```python
from build123d import *

# Parameters (mm, degrees)
F0_R     = 1
F1_DEPTH = 1.5
F3_DEPTH = 1.5
F4_DEPTH = 5
F2_W     = 4.5
F2_H     = 4.5
F2_R     = 1
F5_DEPTH = 3.5


with BuildPart() as f1:
    # F0 (on Top) → F1 (new body)
    with BuildSketch(Plane.XY):
        with BuildLine():
            ThreePointArc((-20.5, 0), (-21.232233047, 1.767766953), (-23, 2.5))
            ThreePointArc((-23, 2.5), (-25.5, 0), (-23, -2.5))
            ThreePointArc((-23, -2.5), (-21.232233047, -1.767766953), (-20.5, 0))
        make_face()
        with Locations((-23, 0)):
            Circle(F0_R, mode=Mode.SUBTRACT)
        with BuildLine():
            Line((23, 2.5), (-23, 2.5))
            ThreePointArc((-23, 2.5), (-21.232233047, 1.767766953), (-20.5, 0))
            ThreePointArc((-20.5, 0), (-21.232233047, -1.767766953), (-23, -2.5))
            Line((-23, -2.5), (23, -2.5))
            ThreePointArc((23, -2.5), (20.5, 0), (23, 2.5))
        make_face()
        with BuildLine():
            ThreePointArc((25.5, 0), (24.767766953, 1.767766953), (23, 2.5))
            ThreePointArc((23, 2.5), (20.5, 0), (23, -2.5))
            ThreePointArc((23, -2.5), (24.767766953, -1.767766953), (25.5, 0))
        make_face()
        with Locations((23, 0)):
            Circle(F0_R, mode=Mode.SUBTRACT)
    extrude(amount=F1_DEPTH)

    # F2 (on face) → F3 (join)
    with BuildSketch(Plane.XZ.offset(2.5)):
        Polygon((8.2, 37.7), (-8.2, 37.7), (-8.2, 33.2), (-12.7, 33.2), (-12.7, 25.25), (-8.2, 25.25), (-8.2, 20.75), (-12.7, 20.75), (-12.7, 13.3), (-8.25, 13.3), (-8.25, 11.8), (-12.7, 11.8), (-12.7, 1.5), (12.7, 1.5), (12.7, 11.8), (8.25, 11.8), (8.25, 13.3), (12.7, 13.3), (12.7, 20.75), (8.2, 20.75), (8.2, 25.25), (12.7, 25.25), (12.7, 33.2), (8.2, 33.2), align=None)
        Polygon((-6.5, 27.5), (-4.5, 27.5), (4.5, 27.5), (6.5, 27.5), (6.5, 16.5), (-6.5, 16.5), align=None, mode=Mode.SUBTRACT)
    extrude(amount=-F3_DEPTH)

    # F2 (on face) → F4 (join)
    with BuildSketch(Plane.XZ.offset(2.5)):
        Polygon((-12.7, 33.2), (-12.7, 37.7), (-8.2, 37.7), (8.2, 37.7), (12.7, 37.7), (12.7, 33.2), (12.7, 25.25), (12.7, 20.75), (12.7, 13.3), (8.25, 13.3), (8.25, 11.8), (12.7, 11.8), (12.7, 1.5), (14.2, 1.5), (14.2, 39.2), (-14.2, 39.2), (-14.2, 1.5), (-12.7, 1.5), (-12.7, 11.8), (-8.25, 11.8), (-8.25, 13.3), (-12.7, 13.3), (-12.7, 20.75), (-12.7, 25.25), align=None)
    extrude(amount=-F4_DEPTH)

    # F2 (on face) → F5 (join)
    with BuildSketch(Plane.XZ.offset(2.5)):
        with Locations((10.45, 35.45)):
            Rectangle(F2_W, F2_H)
        with Locations((10.5, 35.5)):
            Circle(F2_R, mode=Mode.SUBTRACT)
        with Locations((10.45, 23)):
            Rectangle(F2_W, F2_H)
        with Locations((10.5, 23)):
            Circle(F2_R, mode=Mode.SUBTRACT)
        Polygon((-4.5, 18.5), (-4.5, 27.5), (-6.5, 27.5), (-6.5, 16.5), (6.5, 16.5), (6.5, 27.5), (4.5, 27.5), (4.5, 18.5), align=None)
        with Locations((-10.45, 35.45)):
            Rectangle(F2_W, F2_H)
        with Locations((-10.5, 35.5)):
            Circle(F2_R, mode=Mode.SUBTRACT)
        with Locations((-10.45, 23)):
            Rectangle(F2_W, F2_H)
        with Locations((-10.5, 23)):
            Circle(F2_R, mode=Mode.SUBTRACT)
    extrude(amount=-F5_DEPTH)


solid = f1.part
```
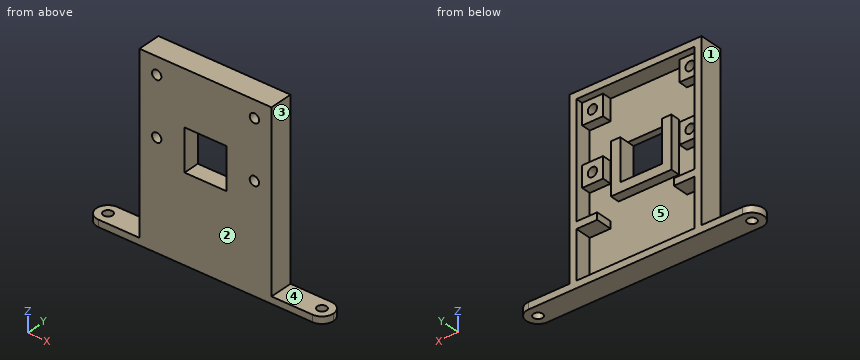
Geometry check sheet. Reference: the model listing, model coordinates, mm. Face numbers are marked on the shaded views. A direction names the side the tool comes from. Give positions to 0.01 mm unless a question says otherwise; leave off trailing zeros. Order: outer loops, then holes, each group sorted by start corner. A loop starts at its lowest first (then second) coordinate and runs counter-clockwise, first axis right, second up. Notation, with made-up numbers: (34.5, 32) -> (67.5, 32) arc R28 cw to (67.5, 68) -> close; hole circle Ø11 at (-14, 52). An arc over 180 degrees is marked (long way). Write each question's results on one line, items separated by ' | '. Start each with the question number.
(1) Sectioned sample at A-A (z = 23). Enter the section's corners in (x, y).
(2) Sectioned sample at C-C (x = 10.5). Enter the section's corners in (y, z), plus the area to 4 significant figures.
(3) Scan lines: line 1 (Z direction, x = -12, y = -0.3); line 2 (Z direction, x = -4, y = 0.65); line 3 (X direction, y = -0.05, z = 17). Record each from-to range of solid material in increasing order.
(4) Sectioned sample at D-D (z = 32). Enter the section's corners in (x, y), plus the area to 3 significant figures.
(5) Gauge pin test, flat ends, axial feed: P1, Ø2.5, axis at x = -10.5, z = 23, coming from the +Y side; P2, Ø1.8, axis at y = 0.5, z = 9, coming from the +X side; P3, Ø1, axis at y = -0.5, z = 22.5, coming from the -X side; P4, Ø1.6, axis at x = 23, y = 0, coming from the -Z side. Record the tip position at first contact, or that the pin passes through.
(6) Access from +Z, -Z, +X, -X, +Y, -Y to the whole of each face (thin tool, end or side, straight path). Record for the marked faces 1 and 2.
(7) Mould release check, pull along X, two halves, no side actions. Record for the marked faces 3, 4 and 5: pulls with the +X half, pulls with the -X half, needs draft (parallel to the pull), parting line crosses it, or undercut.
(8) Sectioned sample at B-B (x = 3.5). Enter the section's corners in (y, z).
Answer below:
1) outline: (-14.2, -2.5) -> (-11.5, -2.5) -> (-11.5, 1) -> (-12.7, 1) -> (-12.7, 2.5) -> (-14.2, 2.5) -> close; (-9.5, -2.5) -> (-4.5, -2.5) -> (-4.5, 1) -> (-6.5, 1) -> (-6.5, -1) -> (-8.2, -1) -> (-8.2, 1) -> (-9.5, 1) -> close; (4.5, -2.5) -> (9.5, -2.5) -> (9.5, 1) -> (8.2, 1) -> (8.2, -1) -> (6.5, -1) -> (6.5, 1) -> (4.5, 1) -> close; (11.5, -2.5) -> (14.2, -2.5) -> (14.2, 2.5) -> (12.7, 2.5) -> (12.7, 1) -> (11.5, 1) -> close
2) outline: (-2.5, 0) -> (2.5, 0) -> (2.5, 1.5) -> (-1, 1.5) -> (-1, 11.8) -> (2.5, 11.8) -> (2.5, 13.3) -> (-1, 13.3) -> (-1, 20.75) -> (1, 20.75) -> (1, 22) -> (-2.5, 22) -> close; (-2.5, 24) -> (1, 24) -> (1, 25.25) -> (-1, 25.25) -> (-1, 33.2) -> (1, 33.2) -> (1, 34.5) -> (-2.5, 34.5) -> close; (-2.5, 36.5) -> (1, 36.5) -> (1, 37.7) -> (2.5, 37.7) -> (2.5, 39.2) -> (-2.5, 39.2) -> close | area: 78.55 mm2
3) line 1: 0 to 1.5, 11.8 to 13.3, 20.75 to 25.25, 33.2 to 39.2 | line 2: 0 to 1.5, 16.5 to 18.5, 37.7 to 39.2 | line 3: -14.2 to -12.7, -6.5 to 6.5, 12.7 to 14.2
4) outline: (-14.2, -2.5) -> (14.2, -2.5) -> (14.2, 2.5) -> (12.7, 2.5) -> (12.7, -1) -> (-12.7, -1) -> (-12.7, 2.5) -> (-14.2, 2.5) -> close | area: 53.1 mm2
5) P1: y = 1 | P2: x = 14.2 | P3: x = -14.2 | P4: through
6) face 1: +Z, -X, +Y, -Y | face 2: +Z, -Z, +X, -X, -Y
7) face 3: pulls with the +X half | face 4: needs draft | face 5: undercut
8) outline: (-2.5, 0) -> (2.5, 0) -> (2.5, 1.5) -> (-1, 1.5) -> (-1, 16.5) -> (1, 16.5) -> (1, 18.5) -> (-2.5, 18.5) -> close; (-2.5, 27.5) -> (-1, 27.5) -> (-1, 37.7) -> (2.5, 37.7) -> (2.5, 39.2) -> (-2.5, 39.2) -> close
